Work out the finished part from the listing and answer in its coordinate system (mm). A direction names the side the tool comes from. Coordinates: 2 decimals unless noted, no trailing zeros. Write each loop counter-clockwise with the first axis right and the second up, starting at its lowest first coordinate (ties: lowest second). Pieces come first, ordered by that corner, then holes. Notation, with made-up numbers: (82.5, -24) - (87.5, -24) arc R31 cw to (87.5, 6) - close; hole circle Ø5 at (61, 19). An arc over 180 degrees is marked (long way). One line per item, written item: value.
Autodesk Inventor part; units mm, degrees
ref_plane "YZ Plane" through (0, 0, 0) normal (1, 0, 0) x (0, 1, 0)
ref_plane "XZ Plane" through (0, 0, 0) normal (0, 1, 0) x (-1, 0, 0)
ref_plane "XY Plane" through (0, 0, 0) normal (0, 0, 1) x (1, 0, 0)
sketch "Sketch1" plane through (0, 0, 0) normal (0, 0, 1) x (1, 0, 0)
  line L0 (-83.5, -75) -> (83.5, -75)
  line L1 (83.5, -75) -> (83.5, 75)
  line L2 (83.5, 75) -> (-83.5, 75)
  line L3 (-83.5, 75) -> (-83.5, -75)
  line L4 (-83.5, -75) -> (83.5, 75) construction
  line L5 (83.5, -75) -> (-83.5, 75) construction
  line L6 (-111.3333, -100) -> (111.3333, -100)
  line L7 (111.3333, -100) -> (111.3333, 100)
  line L8 (111.3333, 100) -> (-111.3333, 100)
  line L9 (-111.3333, 100) -> (-111.3333, -100)
  line L10 (-111.3333, -100) -> (111.3333, 100) construction
  line L11 (111.3333, -100) -> (-111.3333, 100) construction
  point P0 (0, 0)
  dimension "d0" = 167
  dimension "d1" = 150
  dimension "d2" = 200
extrude "Extrusion1" add sketch "Sketch1" along normal blind 6
sketch "Sketch2" plane through (0, 0, 6) normal (0, 0, 1) x (1, 0, 0)
  line L0 (-97.7815, 91.4101) -> (-75.2386, 91.4101) construction
  line L1 (-75.2386, 91.4101) -> (-75.2386, 85.3601) construction
  line L2 (-75.2386, 85.3601) -> (-97.7815, 85.3601) construction
  line L3 (-97.7815, 85.3601) -> (-97.7815, 91.4101) construction
  line L4 (111.3333, -100) -> (111.3333, 100)
  line L5 (111.3333, 100) -> (-111.3333, 100)
  line L6 (-111.3333, 100) -> (-111.3333, -100)
  line L7 (-111.3333, -100) -> (111.3333, -100)
  line L8 (-83.5, -75) -> (-83.5, 75)
  line L9 (-83.5, 75) -> (83.5, 75)
  line L10 (83.5, 75) -> (83.5, -75)
  line L11 (83.5, -75) -> (-83.5, -75)
  point P0 (0, 0)
properties part number "EngravingJigBottom"
Item 1: Section B-B, the plane x = -62 is taken. Determine the outline of the cut face in (y, z).
Evaluation:
outline: (-100, 0) - (-75, 0) - (-75, 6) - (-100, 6) - close; (75, 0) - (100, 0) - (100, 6) - (75, 6) - close
Item 2: Section A-A, the plane y = 54 is taken. Determine the outline of the cut face in (x, z), then the cut area to 3 significant figures.
Evaluation:
outline: (-111.33, 0) - (-83.5, 0) - (-83.5, 6) - (-111.33, 6) - close; (83.5, 0) - (111.33, 0) - (111.33, 6) - (83.5, 6) - close
area: 334 mm2
Item 3: Which of the six approach directions +Z, -Z, +X, -X, +Y, -Y give full straight-line access (tool end or side, diameter ignored) to faces 1 (the face through (83.5, -1, 3)), 2 (the face through (-2, -100, 3))?
Evaluation:
face 1: +Z, -Z
face 2: +Z, -Z, +X, -X, -Y
Item 4: Determine the mould class of faces 3 (the face through (2, 100, 3)), 4 (the face through (-1, -75, 3)), 5 (the face through (111.333, -1, 3)) for opening direction Y: +Y half, -Y half, draft (parallel to the pull), parting line (faces both ways), or undercut.
Evaluation:
face 3: +Y half
face 4: undercut
face 5: draft
Item 5: Consider probe 1 along X at (y, z) = (-22.5, 2.9); probe 2 along Y at (x, z) = (35, 3.7). Determine where each line is inside the solid, lowest interval first.
Evaluation:
probe 1: x = -111.33 to -83.5, 83.5 to 111.33
probe 2: y = -100 to -75, 75 to 100
Item 6: Section C-C, the plane z = 4.75 is taken. Determine the outline of the cut face in (x, y), then the cut area to 3 significant figures.
Evaluation:
outline: (-111.33, -100) - (111.33, -100) - (111.33, 100) - (-111.33, 100) - close; hole (-83.5, -75) - (83.5, -75) - (83.5, 75) - (-83.5, 75) - close
area: 19,500 mm2
